Autodesk Fusion 360 part; units mm, degrees
sketch "Sketch2" plane through (0, 0, 0) normal (1, 0, 0) x (0, 0, -1)
  line L0 (0, 0) -> (-3.2, 0)
  line L1 (-3.2, 0) -> (-3.2, 7)
  line L2 (-3.2, 7) -> (0, 7)
  line L3 (0, 7) -> (0, 0)
  line L4 (-3.2, 0) -> (-26.2, 0)
  line L5 (-26.2, 0) -> (-26.2, 17.8)
  line L6 (-26.2, 17.8) -> (-3.2, 17.8)
  line L7 (-3.2, 17.8) -> (-3.2, 0)
  line L8 (-26.2, 0) -> (-55.2, 0)
  line L9 (-55.2, 0) -> (-55.2, 19.5)
  line L10 (-55.2, 19.5) -> (-26.2, 19.5)
  line L11 (-26.2, 19.5) -> (-26.2, 0)
  line L12 (-55.2, 0) -> (-61.2, 0)
  line L13 (-61.2, 0) -> (-61.2, 6)
  line L14 (-60.2, 6) -> (-55.2, 6)
  line L15 (-55.2, 6) -> (-55.2, 0)
  line L16 (-61.2, 0) -> (-63.4, 0)
  line L17 (-63.4, 0) -> (-63.4, 6)
  line L18 (-63.4, 6) -> (-61.2, 6)
  line L19 (-61.2, 5) -> (-61.2, 0)
  line L20 (-63.4, 0) -> (-78.4, 0)
  line L21 (-78.4, 0) -> (-78.4, 3)
  line L22 (-78.4, 3) -> (-63.4, 3)
  line L23 (-63.4, 3) -> (-63.4, 0)
  line L24 (-60.2, 6) -> (-61.2, 5)
  dimension "d4" = 3.2
  dimension "d6" = 52
  dimension "d7" = 29
  dimension "d8" = 6
  dimension "d9" = 2.2
  dimension "d10" = 23.2
  dimension "d11" = 7
  dimension "d12" = 17.8
  dimension "d13" = 19.5
  dimension "d14" = 6
  dimension "d15" = 6
  dimension "d16" = 3
  dimension "d17" = 1
  dimension "d18" = 1
revolve "Revolve1" add sketch "Sketch2" angle 360 about axis through (0, 0, 63.4) along (0, 0, 1)
sketch "Sketch3" plane through (0, 0, 0) normal (1, 0, 0) x (0, 0, -1)
  line L0 (-78.4, 3) -> (-66.4, 3)
  line L1 (-66.4, 3) -> (-66.4, 2.5)
  line L2 (-66.4, 2.5) -> (-78.4, 2.5)
  line L3 (-78.4, 2.5) -> (-78.4, 3)
  point P0 (-78.4, 3)
  dimension "d20" = 12
  dimension "d21" = 0.5
extrude "Extrude2" cut sketch "Sketch3" along normal through all and the other way through all
sketch "Sketch4" plane through (0, 0, 3.2) normal (0, 0, -1) x (-1, 0, 0)
  circle A0 centre (0, 0) radius 17.8
  circle A1 centre (0, 0) radius 7
  line L0 (2.375, 14.75) -> (-2.375, 14.75)
  line L1 (-2.375, 14.75) -> (-2.375, 15.25)
  line L2 (-2.375, 15.25) -> (2.375, 15.25)
  line L3 (2.375, 15.25) -> (2.375, 14.75)
  line L4 (2.375, 14.75) -> (-2.375, 15.25) construction
  line L5 (-2.375, 14.75) -> (2.375, 15.25) construction
  point P0 (0, 15)
  dimension "d24" = 4.75
  dimension "d25" = 15
  dimension "d26" = 0.5
extrude "Extrude3" add sketch "Sketch4" along normal blind 8 contours L0 L1 L2 L3
mirror "Mirror1" about plane through (0, 0, 0) normal (0, 1, 0) of "Extrude3"
sketch "Sketch5" plane through (0, 15.25, 0) normal (0, 1, 0) x (-1, 0, 0)
  line L0 (2.375, 3.2) -> (-2.375, 3.2)
  line L1 (-2.375, 3.2) -> (-2.375, -4.8)
  line L2 (-2.375, -4.8) -> (2.375, -4.8)
  line L3 (2.375, -4.8) -> (2.375, 3.2)
  circle A0 centre (0, -1.6) radius 1
  dimension "d31" = 2
  dimension "d32" = 3.2
extrude "Extrude4" cut sketch "Sketch5" along normal through all contours A0
chamfer "Chamfer1" distance 0.4 angle 45 4 edges at (-2.375, 15, -4.8) (2.375, 15, -4.8) (2.375, -15, -4.8) (-2.375, -15, -4.8)
sketch "Sketch6" plane through (0, 0, 55.2) normal (0, 0, 1) x (1, 0, 0)
  circle A0 centre (0, 0) radius 6
  circle A1 centre (0, 0) radius 19.5
  circle A2 centre (0, 15.5) radius 1.5
  arc A3 (-1.4982, 15.4274) -> (-14.1097, -6.4162) centre (0, 0) ccw
  dimension "d35" = 3
  dimension "d36" = 31
extrude "Extrude5" cut sketch "Sketch6" against normal blind 3.5 contours A2
thread "Thread1"
pattern_circular "C-Pattern1" count 3 over 360 about axis through (0, 0, 1.75) along (0, 0, 1) of "Extrude5"
equation "d18 = d17"
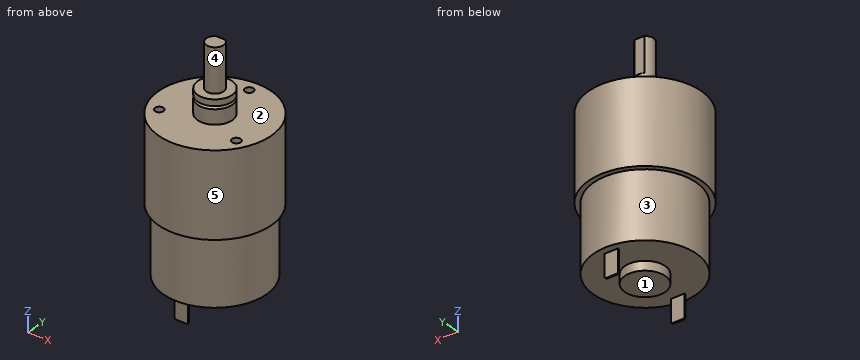
Could you check a few things on this model? Use its own coordinates, in mm. Face numbers are marked on the shaded views. A direction names the side the tool comes from. Coordinates: 2 decimals unless noted, no trailing zeros. Loops run counter-clockwise (first coordinate to the right, second up) from the corner with the lowest first, then second, coordinate; pieces in that order, holes last. Notation, with made-up numbers: M 63.5,-10.5 L 96.5,-10.5 A13 ccw 96.5,2.5 Z; hole C 48.25,49.5 d10. An arc over 180 degrees is marked long. Put each result on its own line as item: value. Start each with the question number.
(1) Suppose I cut it at D-D on x = -11. Please give me the cut outline in (y, z).
(2) I need wall thicknesses on line 1 (Y direction, x = 0, z = 53.4); line 2 (Z direction, x = -13, y = 6); line 3 (Z direction, x = -12, y = 15). Which ranges of each line are inside material? Lowest first, please. Write a range as from..to.
(3) Will these pins go through, and if not, where does the flat tip stop? P1, Ø1.4, axis at x = -0.5, z = 0.5, coming from the -Y side; P2, Ø1.5, axis at x = 0.5, y = -1.5, coming from the -Z side; P3, Ø10, axis at x = -4.5, y = -7.5, coming from the +Z side.
(4) For the marked faces 4 and 5, which set-ups out of +Z, -Z, +X, -X, +Y, -Y let a thin tool reach every point of the face, with its end or its side?
(5) Suppose I cut it at C-C on z = 72.5. Please give me the cut outline in (x, y).
(6) Thinking about a two-plate mould opening in Y: for the marked faces 1, 2 and 3, which applies, pulls with the +Y half, pulls with the -Y half, needs draft (parallel to the pull), parting line crosses it, or undercut?
(7) Suppose I cut it at B-B on x = 10.5. Please give me the cut outline in (y, z), then the cut area to 3 significant figures.
(8) Suppose I cut it at A-A on y = 0. Please give me the cut outline in (x, z), then the cut area to 3 significant figures.
Solutions:
1. outline: M -16.1,26.2 L -13.99,26.2 L -13.99,3.2 L 13.99,3.2 L 13.99,26.2 L 16.1,26.2 L 16.1,55.2 L -16.1,55.2 Z
2. line 1: y = -19.5..14, 17..19.5
2. line 2: z = 3.2..55.2
2. line 3: z = 26.2..55.2
3. P1: stops at y = -15.25
3. P2: stops at z = 0
3. P3: stops at z = 63.4
4. face 4: +Z
4. face 5: +Z, -Z
5. outline: M -1.66,2.5 A3 ccw long 1.66,2.5 Z
6. face 1: undercut
6. face 2: needs draft
6. face 3: parting line crosses it
7. outline: M -16.43,26.2 L -14.37,26.2 L -14.37,3.2 L 14.37,3.2 L 14.37,26.2 L 16.43,26.2 L 16.43,55.2 L -16.43,55.2 Z
7. area: 1,610 mm2
8. outline: M -19.5,26.2 L -17.8,26.2 L -17.8,3.2 L -7,3.2 L -7,0 L 7,0 L 7,3.2 L 17.8,3.2 L 17.8,26.2 L 19.5,26.2 L 19.5,55.2 L 6,55.2 L 6,60.2 L 5,61.2 L 6,61.2 L 6,63.4 L 3,63.4 L 3,78.4 L -3,78.4 L -3,63.4 L -6,63.4 L -6,61.2 L -5,61.2 L -6,60.2 L -6,55.2 L -19.5,55.2 Z
8. area: 2,180 mm2
